Study the drawing (mm; zero at the part's minimum x, y, z) and answer. Give positions to 0.01 mm unless a question says otherwise; leave off trailing zeros. Write each loop counter-clockwise with the first axis right and the second up, starting at its lowest first coordinate (ties: lowest second). Pieces come first, ordered by that corner, then holes. Notation, with made-up numbers: (34, 43) - (85, 43) arc R19 ccw to (85, 61) - close; hole circle Ø6 at (-3.5, 16). An arc over 180 degrees is marked (long way). Write each question's results on one line, items separated by ' | '. Start each with the question number.
Q1. Section C-C (y = 2.25) is taken. Determine the outline of the cut face in (x, z) (3 decimals).
Q2. Section A-A (z = 14) is taken. Determine the outline of the cut face in (x, y) (3 decimals), plus the area to 3 significant figures.
Q3. Section D-D (z = 5) is taken. Determine the outline of the cut face in (x, y) (3 decimals), plus the area to 3 significant figures.
Q4. Section B-B (x = 14) is taken. Determine the outline of the cut face in (y, z) (3 decimals).
Q5. For a pull along X with two mould halves and no side action, classify the marked faces 1, 2 and 3 as pulls with the +X half, pulls with the -X half, needs draft (parallel to the pull), parting line crosses it, or undercut.
Q6. Find the intervals of material crossed by probe 1 along X at (y, z) = (1.6, 14) (3 decimals); probe 2 along X at (y, z) = (2.55, 16.75); probe 3 along X at (y, z) = (1.15, 19.5), in increasing order.
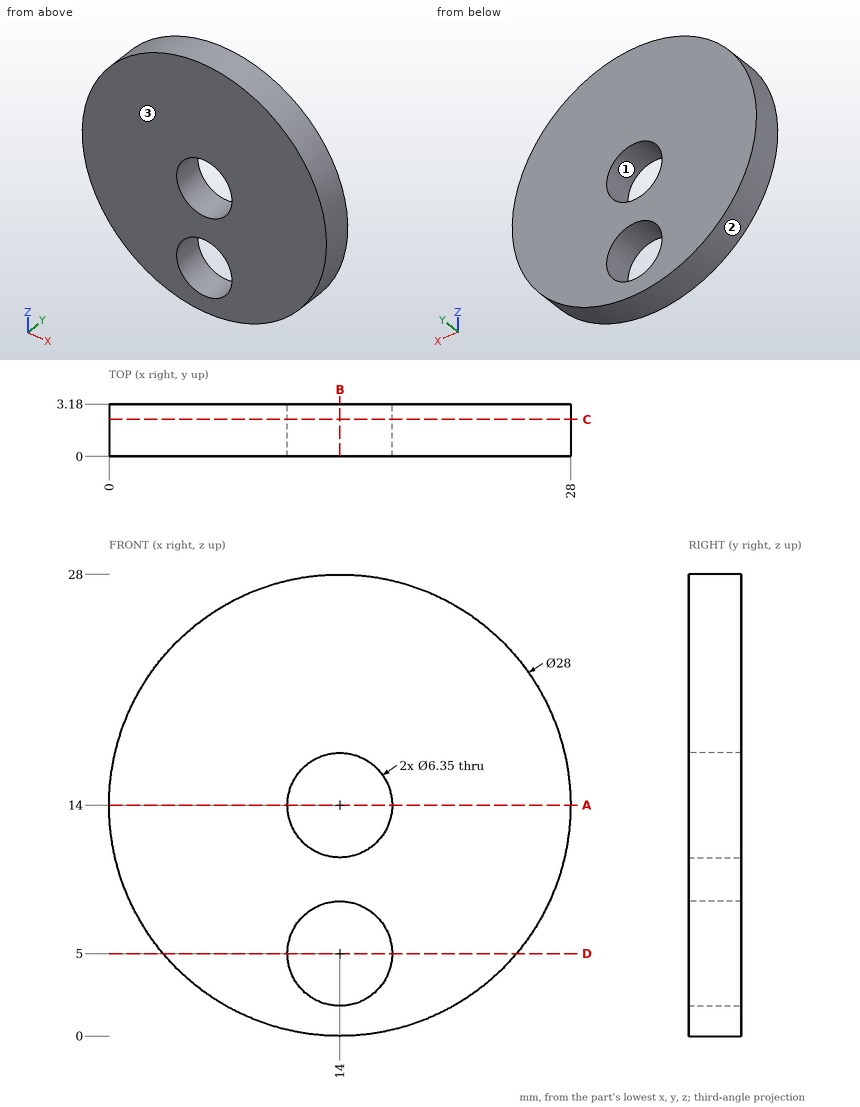
Answers below:
1) outline: circle Ø28 at (14, 14); hole circle Ø6.35 at (14, 5); hole circle Ø6.35 at (14, 14)
2) outline: (0, 0) - (10.825, 0) - (10.825, 3.18) - (0, 3.18) - close; (17.175, 0) - (28, 0) - (28, 3.18) - (17.175, 3.18) - close | area: 68.8 mm2
3) outline: (3.276, 0) - (10.825, 0) - (10.825, 3.18) - (3.276, 3.18) - close; (17.175, 0) - (24.724, 0) - (24.724, 3.18) - (17.175, 3.18) - close | area: 48.0 mm2
4) outline: (0, 0) - (3.18, 0) - (3.18, 1.825) - (0, 1.825) - close; (0, 8.175) - (3.18, 8.175) - (3.18, 10.825) - (0, 10.825) - close; (0, 17.175) - (3.18, 17.175) - (3.18, 28) - (0, 28) - close
5) face 1: undercut | face 2: parting line crosses it | face 3: needs draft
6) probe 1: x = 0 to 10.825, 17.175 to 28 | probe 2: x = 0.27 to 12.41, 15.59 to 27.73 | probe 3: x = 1.13 to 26.87
